```python
from build123d import *

# Parameters (mm, degrees)
CROQUIS1_R              = 18.4
SALIENTE_EXTRUIR1_DEPTH = 54.56
CROQUIS2_R              = 6
SALIENTE_EXTRUIR2_DEPTH = 6
CROQUIS3_R              = 3.5
SALIENTE_EXTRUIR3_DEPTH = 15
CORTAR_EXTRUIR1_START   = -15
CORTAR_EXTRUIR1_DEPTH   = 15
CROQUIS6_R              = 18.42847038
CORTAR_EXTRUIR2_DEPTH   = 30.7
CROQUIS7_R              = 17.4
SALIENTE_EXTRUIR5_DEPTH = 30.7


with BuildPart() as part:
    # Croquis1 → Saliente-Extruir1 (new body)
    with BuildSketch(Plane(origin=(0, 0, 0), x_dir=(1, 0, 0), z_dir=(0, 1, 0))):
        with Locations(Location((0, 0, 0), (0, 0, 270))):
            Circle(CROQUIS1_R)
    extrude(amount=-SALIENTE_EXTRUIR1_DEPTH)

    # Croquis2 → Saliente-Extruir2 (add)
    with BuildSketch(Plane.XZ.offset(54.56)):
        with Locations(Location((0, 6.73, 0), (0, 0, 90))):
            Circle(CROQUIS2_R)
    extrude(amount=SALIENTE_EXTRUIR2_DEPTH)

    # Croquis3 → Saliente-Extruir3 (add)
    with BuildSketch(Plane.XZ.offset(60.56)):
        with Locations(Location((0, 6.73, 0), (0, 0, 270))):
            Circle(CROQUIS3_R)
    extrude(amount=SALIENTE_EXTRUIR3_DEPTH)

    # Croquis4 → Cortar-Extruir1 (cut)
    with BuildSketch(Plane(origin=(0, -75.56, 0), x_dir=(-1, 0, 0), z_dir=(0, -1, 0)).offset(CORTAR_EXTRUIR1_START)):
        with BuildLine():
            Line((2.449489743, -4.23), (-2.449489743, -4.23))
            ThreePointArc((-2.449489743, -4.23), (0, -3.23), (2.449489743, -4.23))
        make_face()
    extrude(amount=CORTAR_EXTRUIR1_DEPTH, mode=Mode.SUBTRACT)

    # Croquis6 → Cortar-Extruir2 (cut)
    with BuildSketch(Plane(origin=(0, 0, 0), x_dir=(1, 0, 0), z_dir=(0, 1, 0))):
        Circle(CROQUIS6_R)
    extrude(amount=-CORTAR_EXTRUIR2_DEPTH, mode=Mode.SUBTRACT)

    # Croquis7 → Saliente-Extruir5 (add)
    with BuildSketch(Plane(origin=(0, -30.7, 0), x_dir=(1, 0, 0), z_dir=(0, 1, 0))):
        with Locations(Location((0, 0, 0), (0, 0, 270))):
            Circle(CROQUIS7_R)
    extrude(amount=SALIENTE_EXTRUIR5_DEPTH)


solid = part.part
```
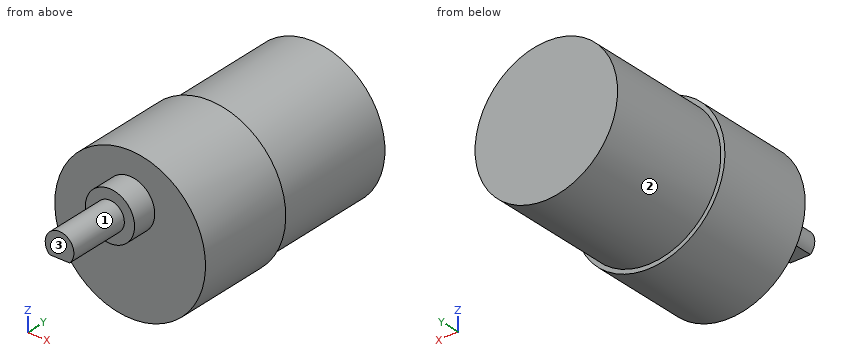
Could you check a few things on this model? Use its own coordinates, in mm. Face numbers are marked on the shaded views. A direction names the side the tool comes from. Round coordinates to 2 decimals unless told otherwise and drop trailing zeros. Order: outer loops, then holes, each group sorted by start corner. A loop starts at its lowest first (then second) coordinate and runs counter-clockwise, first axis right, second up. Notation, with made-up numbers: M -31.75,47.5 L -0.75,47.5 A12 ccw -0.75,55.5 Z; hole C -0.75,28.25 d8. An arc over 180 degrees is marked long. One line per question, with ' | ' between items. Start each with the question number.
(1) Suppose I cut it at D-D on z = -11. List the corners of the cut face in (x, y) for me, then the cut area to 3 significant figures.
(2) Please list where these lines run through material, in increasing order: line 1 along Y through (x, z) = (10, 4.5); line 2 along Y through (x, z) = (1.5, 4); line 3 along Z through (x, y) = (0.5, -25.5).
(3) Suppose I cut it at B-B on z = 6.73. List the corners of the cut face in (x, y) for me, then the cut area to 3 significant figures.
(4) Suppose I cut it at A-A on x = 0. List the corners of the cut face in (y, z) for me, then the cut area to 3 significant figures.
(5) For the marked faces 1, 2 and 3, which set-ups out of +Z, -Z, +X, -X, +Y, -Y let a thin tool reach every point of the face, with its end or its side?
(6) Suppose I cut it at C-C on y = -53. List the corners of the cut face in (x, z) for me.
(7) For P1, Ø8, axis at x = -5, y = -45, coming from the +Z side; P2, Ø5, axis at x = 4, y = -27, coming from the +Z side; P3, Ø1, axis at x = 9, y = -38.5, coming from the +Z side, each with a flat end and sliding along its axis, tell me the tip position at first contact or that it passes through.
Geometry results:
1) outline: M -14.75,-54.56 L 14.75,-54.56 L 14.75,-30.7 L 13.48,-30.7 L 13.48,0 L -13.48,0 L -13.48,-30.7 L -14.75,-30.7 Z | area: 1,530 mm²
2) line 1: -54.56 to 0 | line 2: -60.56 to 0 | line 3: -17.39 to 17.39
3) outline: M -17.13,-54.56 L -6,-54.56 L -6,-60.56 L -3.5,-60.56 L -3.5,-75.56 L 3.5,-75.56 L 3.5,-60.56 L 6,-60.56 L 6,-54.56 L 17.13,-54.56 L 17.13,-30.7 L 16.05,-30.7 L 16.05,0 L -16.05,0 L -16.05,-30.7 L -17.13,-30.7 Z | area: 1,980 mm²
4) outline: M -75.56,4.23 L -60.56,4.23 L -60.56,0.73 L -54.56,0.73 L -54.56,-18.4 L -30.7,-18.4 L -30.7,-17.4 L 0,-17.4 L 0,17.4 L -30.7,17.4 L -30.7,18.4 L -54.56,18.4 L -54.56,12.73 L -60.56,12.73 L -60.56,10.23 L -75.56,10.23 Z | area: 2,110 mm²
5) face 1: -Y | face 2: +Y | face 3: +Z, -Z, +X, -X, -Y
6) outline: C 0,0 d36.8
7) P1: z = 18.37 | P2: z = 17.34 | P3: z = 16.32
